Verification items for this drawing (mm, ordinates from the low corner). A direction names the side the tool comes from. Round coordinates to 2 decimals unless told otherwise and drop trailing zeros. Loops run counter-clockwise (first coordinate to the right, second up) from the corner with the lowest first, then second, coordinate; pieces in that order, holes last. Notation, with made-up numbers: M 28,44 L 71,44 A33 cw 71,74 Z; hole C 62.25,48.25 d9. An arc over 180 degrees is marked long. One line per item, written item: value.
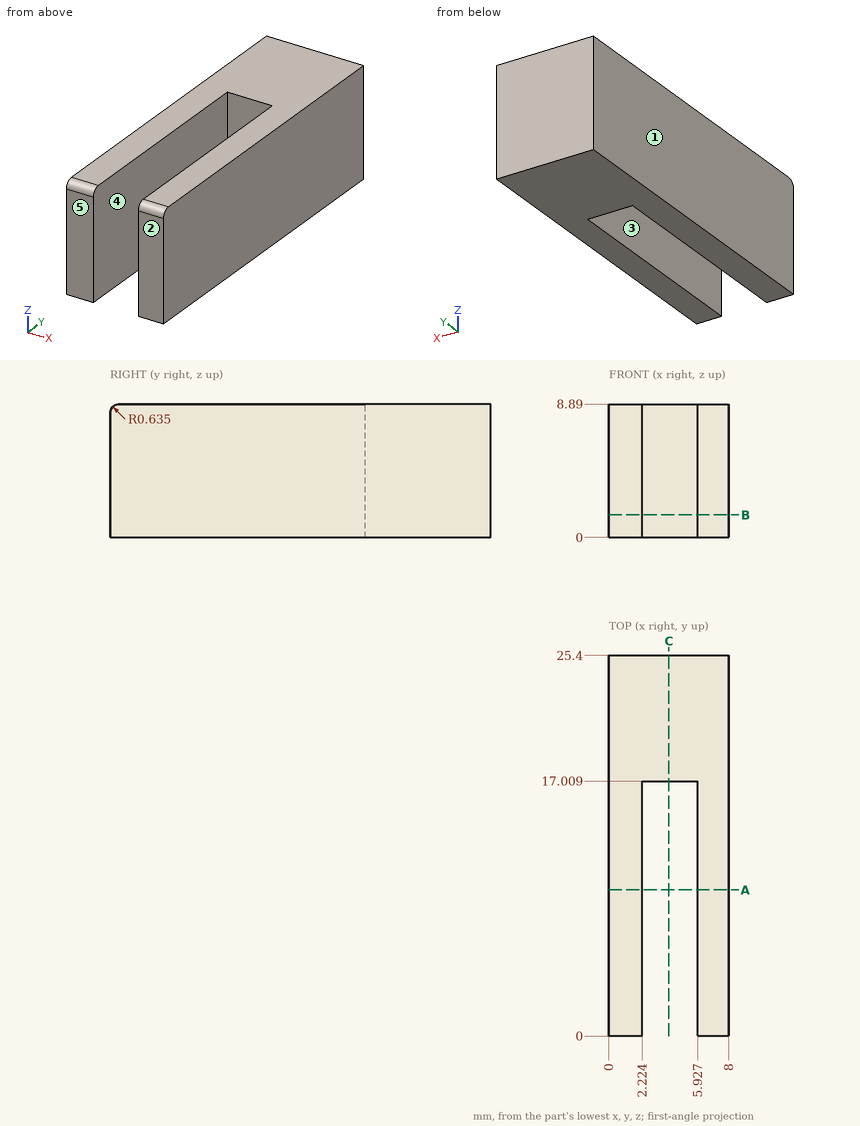
(1) Depth check by flat-ended pin: pin 1 Ø2 at (x, z) = (4, 4.5) entering from -Y; pin 2 Ø4 at (x, y) = (5, 8) entering from +Z. Enter the tip coordinate at first touch or a pass-through.
Completed:
pin 1: stops at y = 17.01
pin 2: stops at z = 8.89
(2) Sectioned sample at C-C on x = 4. Enter the section's corners in (y, z), and give its area (3 significant figures).
Completed:
outline: M 17.01,0 L 25.4,0 L 25.4,8.89 L 17.01,8.89 Z
area: 74.6 mm^2
(3) Tool access check on the marked faces 4 and 5. Record the directions out of +Z, -Z, +X, -X, +Y, -Y that give a thin tool (end or side, any length) a straight path to the whole face; none if there is none.
Completed:
face 4: +Z, -Z, -Y
face 5: +Z, -Z, +X, -X, -Y
(4) Mould release check, pull along X, two halves, no side actions. Record for the marked faces 1, 2 and 3: +X half, -X half, draft (parallel to the pull), parting line (faces both ways), or undercut.
Completed:
face 1: -X half
face 2: draft
face 3: undercut
(5) Sectioned sample at B-B on z = 1.5. Enter the section's corners in (x, y), and give its area (3 significant figures).
Completed:
outline: M 0,0 L 2.22,0 L 2.22,17.01 L 5.93,17.01 L 5.93,0 L 8,0 L 8,25.4 L 0,25.4 Z
area: 140 mm^2
(6) Thickness scan on L1, parallel to X at y = 7.75, z = 2; L2, parallel to Y at x = 4.25, z = 6.75. Record the ranges inside material, lowest first. Write a range as from..to.
Completed:
L1: x = 0..2.22, 5.93..8
L2: y = 17.01..25.4
(7) Sectioned sample at A-A on y = 9.75. Enter the section's corners in (x, z).
Completed:
outline: M 0,0 L 2.22,0 L 2.22,8.89 L 0,8.89 Z; M 5.93,0 L 8,0 L 8,8.89 L 5.93,8.89 Z
